Read the model definition and answer for the solid it produces. Units are mm, in the model's axes. Face numbers are marked on the shaded views. Coordinates: 2 decimals unless noted, no trailing zeros. Write each loop counter-clockwise with the first axis right and the second up, starting at its lowest first coordinate (ties: lowest second). Pieces come first, ordered by that corner, then holes. Notation, with made-up numbers: (1, 20.25) -> (11, 20.25) arc R14 ccw to (11, 30.25) -> close; hole circle Ø5 at (76, 69). An arc over 180 degrees is marked (long way). One line per item, written item: value. Start each with the question number.
1. Find section D-D, the plane x = 16. Write down the section's boundary in (y, z), and give its area (3 significant figures).
2. For a pull along Y with two mould halves and no side action, classify the marked faces 1, 2, 3 and 4 as pulls with the +Y half, pulls with the -Y half, needs draft (parallel to the pull), parting line crosses it, or undercut.
3. Given P1, Ø10, axis at x = 16, y = 16, coming from the -Z side; P2, Ø1.9, axis at x = 15.5, y = 15.5, coming from the +Z side, each flat-ended and moving along its own axis, determine where each tip first touches the part or whether it passes through.
4. Find section A-A, the plane x = 0. Write down the section's boundary in (y, z), and give its area (3 significant figures).
5. Consider line 1 along Y through (x, z) = (-16.5, 6.5); line 2 along Y through (x, z) = (16, 18.9); line 3 along Z through (x, y) = (-16, 13). Determine where each line is inside the solid, lowest interval first.
6. Find section C-C, the plane z = 18. Write down the section's boundary in (x, y), and give its area (3 significant figures).
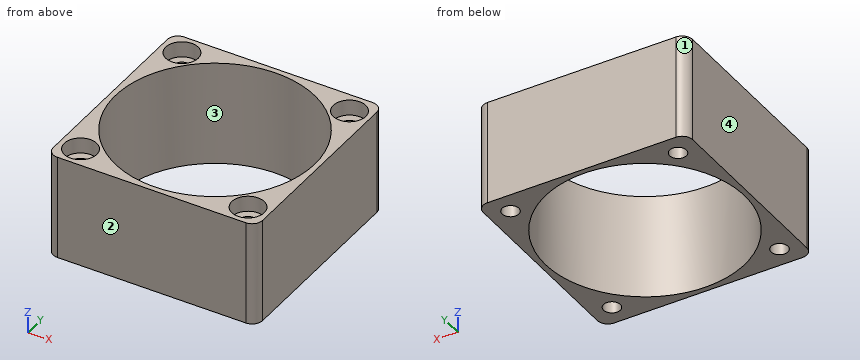
```python
from build123d import *

# Parameters (mm, degrees)
SKETCH1_W           = 40
SKETCH1_H           = 40
BOSS_EXTRUDE1_DEPTH = 20
SKETCH2_R           = 19
SKETCH2_R_2         = 1.6
CUT_EXTRUDE1_DEPTH  = 21
FILLET1_R           = 2
SKETCH3_R           = 3.1
CUT_EXTRUDE2_DEPTH  = 3


with BuildPart() as part:
    # Sketch1 → Boss-Extrude1 (new body)
    with BuildSketch(Plane.XY):
        Rectangle(SKETCH1_W, SKETCH1_H)
    extrude(amount=BOSS_EXTRUDE1_DEPTH)

    # Sketch2 → Cut-Extrude1 (cut, through all)
    with BuildSketch(Plane.XY.offset(20)):
        Circle(SKETCH2_R)
        with Locations((-16, 16)):
            Circle(SKETCH2_R_2)
        with Locations((16, 16)):
            Circle(SKETCH2_R_2)
        with Locations((16, -16)):
            Circle(SKETCH2_R_2)
        with Locations((-16, -16)):
            Circle(SKETCH2_R_2)
    extrude(amount=-CUT_EXTRUDE1_DEPTH, mode=Mode.SUBTRACT)

    # Fillet1
    fillet1_edges = [part.edges().sort_by_distance(p)[0] for p in [
        (20, -20, 10),
        (-20, -20, 10),
        (-20, 20, 10),
        (20, 20, 10),
    ]]
    fillet(fillet1_edges, radius=FILLET1_R)

    # Sketch3 → Cut-Extrude2 (cut)
    with BuildSketch(Plane.XY.offset(20)):
        with Locations((-16, -16)):
            Circle(SKETCH3_R)
        with Locations((16, -16)):
            Circle(SKETCH3_R)
        with Locations((16, 16)):
            Circle(SKETCH3_R)
        with Locations((-16, 16)):
            Circle(SKETCH3_R)
    extrude(amount=-CUT_EXTRUDE2_DEPTH, mode=Mode.SUBTRACT)


solid = part.part
```
Answer block:
1. outline: (-20, 0) -> (-17.6, 0) -> (-17.6, 17) -> (-19.1, 17) -> (-19.1, 20) -> (-20, 20) -> close; (-14.4, 0) -> (-10.25, 0) -> (-10.25, 20) -> (-12.9, 20) -> (-12.9, 17) -> (-14.4, 17) -> close; (10.25, 0) -> (14.4, 0) -> (14.4, 17) -> (12.9, 17) -> (12.9, 20) -> (10.25, 20) -> close; (17.6, 0) -> (20, 0) -> (20, 20) -> (19.1, 20) -> (19.1, 17) -> (17.6, 17) -> close
1. area: 244 mm2
2. face 1: pulls with the +Y half
2. face 2: pulls with the -Y half
2. face 3: undercut
2. face 4: needs draft
3. P1: stops at z = 0
3. P2: stops at z = 17
4. outline: (-20, 0) -> (-19, 0) -> (-19, 20) -> (-20, 20) -> close; (19, 0) -> (20, 0) -> (20, 20) -> (19, 20) -> close
4. area: 40.0 mm2
5. line 1: y = -20 to -17.52, -14.48 to -9.42, 9.42 to 14.48, 17.52 to 20
5. line 2: y = -20 to -19.1, -12.9 to -10.25, 10.25 to 12.9, 19.1 to 20
5. line 3: z = 0 to 17
6. outline: (-20, -18) arc R2 ccw to (-18, -20) -> (18, -20) arc R2 ccw to (20, -18) -> (20, 18) arc R2 ccw to (18, 20) -> (-18, 20) arc R2 ccw to (-20, 18) -> close; hole circle Ø6.2 at (-16, -16); hole circle Ø6.2 at (-16, 16); hole circle Ø38 at (0, 0); hole circle Ø6.2 at (16, -16); hole circle Ø6.2 at (16, 16)
6. area: 342 mm2
